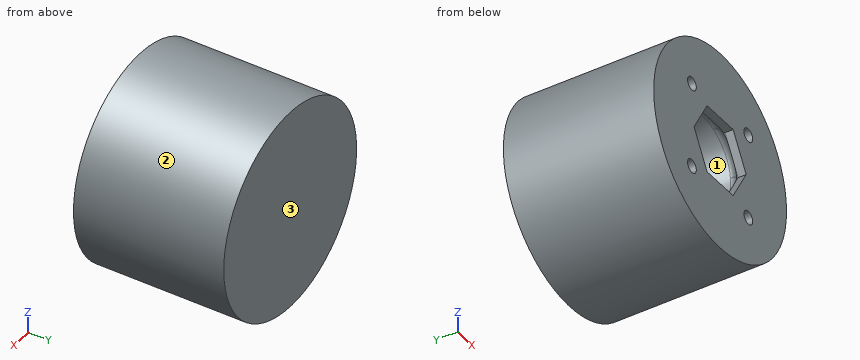
```python
from build123d import *

# Parameters (mm, degrees)
ENL_V_MAT_EXTRU_1_DEPTH = 4
CONG_1_R                = 2
ESQUISSE3_R             = 1.65
ENL_V_MAT_EXTRU_2_DEPTH = 20


with BuildPart() as part:
    # Esquisse1 → Révolution2 (revolve)
    with BuildSketch(Plane.XY, mode=Mode.PRIVATE) as r_volution2_sk:
        with BuildLine():
            Line((-7.394355414, 1.254395478), (-11, -20))
            Line((-11, -20), (-8, -20))
            Line((-8, -20), (-8, -22))
            Line((-8, -22), (-25, -22))
            Line((-25, -22), (-25, -20))
            Line((-25, -20), (-25, 15))
            Line((-25, 15), (0, 15))
            Line((0, 15), (0, 7.5))
            ThreePointArc((0, 7.5), (-4.839526522, 5.729658196), (-7.394355414, 1.254395478))
        make_face()
    revolve(r_volution2_sk.sketch.rotate(Axis((0, 7.5, 0), (0, 1, 0)), 180), axis=Axis((0, 7.5, 0), (0, 1, 0)))

    # Esquisse2 → Enlèv. mat.-Extru.1 (cut)
    with BuildSketch(Plane.XZ.offset(22)):
        Polygon((9.814954576, 0), (4.907477288, 8.5), (-4.907477288, 8.5), (-9.814954576, 0), (-4.907477288, -8.5), (4.907477288, -8.5), align=None)
    extrude(amount=-ENL_V_MAT_EXTRU_1_DEPTH, mode=Mode.SUBTRACT)

    # Congé1
    # the kernel refuses this fillet: 2 mm, written as the material it adds along each edge
    with BuildSketch(Plane(origin=(0, -20, 0), x_dir=(1, 0, 0), z_dir=(0, 0, 1))) as cong_1_piece_1_section:
        with BuildLine():
            CenterArc((11 - CONG_1_R * 1.1839294959, CONG_1_R), CONG_1_R, 270, 99.628125236)
            Line((11 - CONG_1_R * 1.1839294959, 0), (11, 0))
            Line((11, 0), (11 - CONG_1_R * 0.198015440727, CONG_1_R * 1.16725273035))
        make_face()
    cong_1_piece_1 = revolve(axis=Axis((0, -20, 0), (0, 1, 0)), mode=Mode.PRIVATE)
    cong_1_piece_1 = split(cong_1_piece_1, bisect_by=Plane(origin=(10.002736097, -19.349469748, 0.325247134), z_dir=(0.8660254037844389, 0, -0.49999999999999956)), keep=Keep.TOP, mode=Mode.PRIVATE)
    with BuildSketch(Plane(origin=(0, -20, 0), x_dir=(1, 0, 0), z_dir=(0, 0, 1))) as cong_1_piece_2_section:
        with BuildLine():
            CenterArc((11 - CONG_1_R * 1.1839294959, CONG_1_R), CONG_1_R, 270, 99.628125236)
            Line((11 - CONG_1_R * 1.1839294959, 0), (11, 0))
            Line((11, 0), (11 - CONG_1_R * 0.198015440727, CONG_1_R * 1.16725273035))
        make_face()
    cong_1_piece_2 = revolve(axis=Axis((0, -20, 0), (0, 1, 0)), mode=Mode.PRIVATE)
    cong_1_piece_2 = split(cong_1_piece_2, bisect_by=Plane(origin=(7.361215688, -19.472047685, 4.250000423), z_dir=(0.8660254037844387, 0, 0.5000000000000003)), keep=Keep.TOP, mode=Mode.PRIVATE)
    with BuildSketch(Plane(origin=(0, -20, 0), x_dir=(1, 0, 0), z_dir=(0, 0, 1))) as cong_1_piece_3_section:
        with BuildLine():
            CenterArc((11 - CONG_1_R * 1.1839294959, CONG_1_R), CONG_1_R, 270, 99.628125236)
            Line((11 - CONG_1_R * 1.1839294959, 0), (11, 0))
            Line((11, 0), (11 - CONG_1_R * 0.198015440727, CONG_1_R * 1.16725273035))
        make_face()
    cong_1_piece_3 = revolve(axis=Axis((0, -20, 0), (0, 1, 0)), mode=Mode.PRIVATE)
    cong_1_piece_3 = split(cong_1_piece_3, bisect_by=Plane(origin=(-2.9e-08, -19.472047136, -8.5), z_dir=(0, 0, -1)), keep=Keep.TOP, mode=Mode.PRIVATE)
    with BuildSketch(Plane(origin=(0, -20, 0), x_dir=(1, 0, 0), z_dir=(0, 0, 1))) as cong_1_piece_4_section:
        with BuildLine():
            CenterArc((11 - CONG_1_R * 1.1839294959, CONG_1_R), CONG_1_R, 270, 99.628125236)
            Line((11 - CONG_1_R * 1.1839294959, 0), (11, 0))
            Line((11, 0), (11 - CONG_1_R * 0.198015440727, CONG_1_R * 1.16725273035))
        make_face()
    cong_1_piece_4 = revolve(axis=Axis((0, -20, 0), (0, 1, 0)), mode=Mode.PRIVATE)
    cong_1_piece_4 = split(cong_1_piece_4, bisect_by=Plane(origin=(2.9e-08, -19.472047136, 8.5), z_dir=(0, 0, 1)), keep=Keep.TOP, mode=Mode.PRIVATE)
    with BuildSketch(Plane(origin=(0, -20, 0), x_dir=(1, 0, 0), z_dir=(0, 0, 1))) as cong_1_piece_5_section:
        with BuildLine():
            CenterArc((11 - CONG_1_R * 1.1839294959, CONG_1_R), CONG_1_R, 270, 99.628125236)
            Line((11 - CONG_1_R * 1.1839294959, 0), (11, 0))
            Line((11, 0), (11 - CONG_1_R * 0.198015440727, CONG_1_R * 1.16725273035))
        make_face()
    cong_1_piece_5 = revolve(axis=Axis((0, -20, 0), (0, 1, 0)), mode=Mode.PRIVATE)
    cong_1_piece_5 = split(cong_1_piece_5, bisect_by=Plane(origin=(-7.361215946, -19.472047136, -4.249999975), z_dir=(-0.8660254037844387, 0, -0.5000000000000001)), keep=Keep.TOP, mode=Mode.PRIVATE)
    with BuildSketch(Plane(origin=(0, -20, 0), x_dir=(1, 0, 0), z_dir=(0, 0, 1))) as cong_1_piece_6_section:
        with BuildLine():
            CenterArc((11 - CONG_1_R * 1.1839294959, CONG_1_R), CONG_1_R, 270, 99.628125236)
            Line((11 - CONG_1_R * 1.1839294959, 0), (11, 0))
            Line((11, 0), (11 - CONG_1_R * 0.198015440727, CONG_1_R * 1.16725273035))
        make_face()
    cong_1_piece_6 = revolve(axis=Axis((0, -20, 0), (0, 1, 0)), mode=Mode.PRIVATE)
    cong_1_piece_6 = split(cong_1_piece_6, bisect_by=Plane(origin=(-7.361215918, -19.472047136, 4.250000025), z_dir=(-0.8660254037844387, 0, 0.4999999999999999)), keep=Keep.TOP, mode=Mode.PRIVATE)
    add([cong_1_piece_1, cong_1_piece_2, cong_1_piece_3, cong_1_piece_4, cong_1_piece_5, cong_1_piece_6])

    # Esquisse3 → Enlèv. mat.-Extru.2 (cut)
    with BuildSketch(Plane.XZ.offset(22)):
        with Locations((10.606601718, -10.606601718)):
            Circle(ESQUISSE3_R)
        with Locations((-10.606601718, -10.606601718)):
            Circle(ESQUISSE3_R)
        with Locations((-10.606601718, 10.606601718)):
            Circle(ESQUISSE3_R)
        with Locations((10.606601718, 10.606601718)):
            Circle(ESQUISSE3_R)
    extrude(amount=-ENL_V_MAT_EXTRU_2_DEPTH, mode=Mode.SUBTRACT)


solid = part.part
```
Verification items for the finished model (mm, model axes). Face numbers are marked on the shaded views. Coordinates: 2 decimals unless noted, no trailing zeros. Write each loop counter-clockwise with the first axis right and the second up, starting at its lowest first coordinate (ties: lowest second). Pieces come first, ordered by that corner, then holes. Notation, with made-up numbers: (-3, 82.5) - (55, 82.5) arc R5 ccw to (55, 90.5) - close; hole circle Ø10 at (-30.5, 33.25). An arc over 180 degrees is marked (long way). Write item = value, one per line.
Q1. Mould release check, pull along Z, two halves, no side actions. Record for the marked faces 1, 2 and 3: released by +Z, released by -Z, zero draft, split by the parting line, or undercut.
Answer:
face_1 = undercut
face_2 = split by the parting line
face_3 = zero draft
Q2. Go/stop test with flat-tipped pins: pin 1 Ø4.5 at (x, z) = (-10.61, -10.61) entering from -Y; pin 2 Ø1.2 at (x, y) = (1.5, -20.5) entering from +Z; pin 3 Ø1.7 at (x, z) = (-11, 11) entering from -Y; pin 4 Ø2 at (y, z) = (-1.5, -14) entering from -X. Record where each tip stops, or that it passes through.
Answer:
pin_1 = -22
pin_2 = 24.98
pin_3 = -2
pin_4 = -21.35
Q3. Cross-section at A-A (x = 0). Enter the section's corners in (y, z).
Answer:
outline = (-22, -25) - (15, -25) - (15, 25) - (-22, 25) - (-22, 8.5) - (-20, 8.5) - (-20, 8.63) arc R2 cw to (-17.67, 10.6) - (1.25, 7.39) arc R7.5 cw to (1.25, -7.39) - (-17.67, -10.6) arc R2 cw to (-20, -8.63) - (-20, -8.5) - (-22, -8.5) - close
Q4. Cross-section at C-C (z = 20). Enter the section's corners in (x, y).
Answer:
outline = (-15, -22) - (15, -22) - (15, 15) - (-15, 15) - close
Q5. Material ranges on L1, parallel to X at y = -8, z = 11; L2, parallel to Z at x = 10, y = -5.5; L3, parallel to Z at x = -12, y = -18.5, recorded low to high. Write a range as from..to.
Answer:
L1 = -22.45..-12.21, -9..9, 12.21..22.45
L2 = -22.91..-12.14, -9.07..9.07, 12.14..22.91
L3 = -21.93..-11.49, -9.72..9.72, 11.49..21.93
Q6. Cross-section at B-B (y = -13). Give the number of separate pieces and of enclosed holes in the cut face, plus the area to 3 significant figures.
Answer:
separate_pieces = 1
enclosed_holes = 5
area = 1,630 mm²
Q7. Cross-section at D-D (y = 12.5). Enter the section's corners in (x, z), plus the area to 3 significant figures.
Answer:
outline = circle Ø50 at (0, 0)
area = 1,960 mm²
